```python
from build123d import *

# Parameters (mm, degrees)
F1_DEPTH = 63.5
F0_W     = 32.3452991128
F0_H     = 19.05
F0_H_2   = 8.5344
F2_DEPTH = 25.4


with BuildPart() as f1:
    # F0 (on Front) → F1 (new body, symmetric)
    with BuildSketch(Plane.XZ):
        Polygon((-41.275, 9.525), (-41.275, -9.525), (41.275, -9.525), (41.275, 9.525), (22.225, 9.525), align=None)
    extrude(amount=F1_DEPTH, both=True)

    # F0 (on Front) → F2 (join)
    with BuildSketch(Plane.XZ):
        Polygon((-41.275, 9.525), (-41.275, -9.525), (41.275, -9.525), (41.275, 9.525), (22.225, 9.525), align=None)
        with BuildLine():
            add(Edge.make_bspline(
                [(-41.275, 9.525), (-42.1845465899, 39.2021462321), (-14.9138346314, 68.9535290003), (46.3458457894, 60.212033385)],
                knots=[0, 0, 0, 0, 101.22543144, 101.22543144, 101.22543144, 101.22543144], degree=3))
            Line((-41.275, 9.525), (22.225, 9.525))
            Line((22.225, 9.525), (22.225, 27.0002))
            ThreePointArc((22.225, 27.0002), (28.891455179, 47.5236078456), (46.3458457894, 60.212033385))
        make_face()
        with BuildLine():
            Line((22.225, 9.525), (41.275, 9.525))
            Line((41.275, 9.525), (41.275, 27.0002))
            ThreePointArc((41.275, 27.0002), (45.9246798487, 38.2255201513), (57.15, 42.8752))
            Line((57.15, 42.8752), (60.325, 42.8752))
            Line((60.325, 42.8752), (60.325, 61.9252))
            Line((60.325, 61.9252), (57.15, 61.9252))
            ThreePointArc((57.15, 61.9252), (51.6804321913, 61.4942495301), (46.3458457894, 60.212033385))
            ThreePointArc((46.3458457894, 60.212033385), (28.891455179, 47.5236078456), (22.225, 27.0002))
            Line((22.225, 27.0002), (22.225, 9.525))
        make_face()
        with Locations((76.4976495564, 52.4002)):
            Rectangle(F0_W, F0_H)
        Polygon((60.325, 62.9158), (60.325, 61.9252), (92.6702991128, 61.9252), (92.6702991128, 42.8752), (92.6702991128, 34.3408), (111.125, 34.3408), (111.125, 62.9158), align=None)
        with Locations((76.4976495564, 38.608)):
            Rectangle(F0_W, F0_H_2)
    extrude(amount=F2_DEPTH)


solid = f1.part
```
For this review, take the finished solid that the model builds, in its own axes (mm). A direction names the side the tool comes from. Coordinates: 2 decimals unless noted, no trailing zeros. Write each loop counter-clockwise with the first axis right and the second up, starting at its lowest first coordinate (ties: lowest second). Pieces come first, ordered by that corner, then holes. Notation, with made-up numbers: (54.25, -29.75) - (71.25, -29.75) arc R15 cw to (71.25, -8.75) - close; hole circle Ø2 at (32.25, 49). An arc over 180 degrees is marked (long way). Put each result on its own line as item: value.
1. For pin 1 (12 mm diameter, centred on x = 95.5, z = 34.5, fed in from -Y); pin 2 (3 mm diameter, centred on x = -7.5, z = 40.5, fed in from +Y); pin 3 (10 mm diameter, centred on x = 46, y = 44, fed in from +Z) (3 decimals), all flat-tipped, find the tip position at first contact; note any pin that passes through.
Values found:
pin 1: y = -25.4
pin 2: y = 0
pin 3: z = 9.525
2. Add section B-B, the plane z = -1.5. Give the boundary of the cut face in (x, y) (3 decimals), then the cut area to 3 significant figures.
Values found:
outline: (-41.275, -63.5) - (41.275, -63.5) - (41.275, 63.5) - (-41.275, 63.5) - close
area: 10,500 mm²
3. Wall thickness on probe 1 along Y at (x, z) = (29, 40); probe 2 along X at (y, z) = (-28, -3) (3 decimals); probe 3 along Z at (x, y) = (-27.5, -44) (3 decimals): over which ranges is each line inside the solid? List them lowest first.
Values found:
probe 1: -25.4 to 0
probe 2: -41.275 to 41.275
probe 3: -9.525 to 9.525
4. Machinability: for faces 1 (the flat face through (1, 31, 9.525)), 2 (the flat face through (59, -13, 61.925)), 3 (the flat face through (41.275, -1, 4)), 4 (the flat face through (1, -45, 9.525)), 5 (the flat face through (60.325, -13, 39)), which of the approach directions +Z, -Z, +X, -X, +Y, -Y give a long, thin tool a straight path to every point of the face, cutting with its end or side? Answer none if there is none.
Values found:
face 1: +Z, +X, -X, +Y
face 2: +Z, -X, +Y, -Y
face 3: -Z, +X, +Y, -Y
face 4: +Z, +X, -X, -Y
face 5: -Z, +Y, -Y
5. Mouldability with a two-part tool opening along X and no side actions: class faces 6 (the flat face through (111.125, -13, 48)), 7 (the cylindrical face through (51.756, -12.522, 61.506)), 8 (the flat face through (33, -25.4, 40)) as released by +X, released by -X, zero draft, split by the parting line, or undercut.
Values found:
face 6: released by +X
face 7: undercut
face 8: zero draft
6. Add section A-A, the plane y = 5.5. Give the boundary of the cut face in (x, z) (3 decimals).
Values found:
outline: (-41.275, -9.525) - (41.275, -9.525) - (41.275, 9.525) - (-41.275, 9.525) - close
